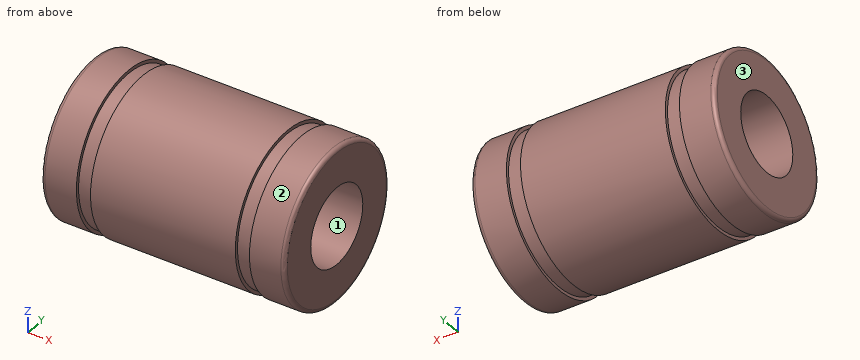
from build123d import *

# Parameters (mm, degrees)
F3_R = 0.3


with BuildPart() as f2:
    # F1 (on Front) → F2 (revolve)
    with BuildSketch(Plane.XZ):
        Polygon((-9.5, 6), (-9.5, 3), (9.5, 3), (9.5, 6), (6.75, 6), (6.75, 5.75), (5.65, 5.75), (5.65, 6), (-5.65, 6), (-5.65, 5.75), (-6.75, 5.75), (-6.75, 6), align=None)
    revolve(axis=Axis((0, 0, 0), (1, 0, 0)))

    # F3
    f3_edges = [f2.edges().sort_by_distance(p)[0] for p in [
        (-9.5, 0, -6),
        (9.5, 0, -6),
    ]]
    fillet(f3_edges, radius=F3_R)


solid = f2.part
Can you work these out from the model? Positions are in its coordinate system, mm. Face numbers are marked on the shaded views. Coordinates: 2 decimals unless noted, no trailing zeros. Order: outer loops, then holes, each group sorted by start corner. A loop starts at its lowest first (then second) coordinate and runs counter-clockwise, first axis right, second up. Notation, with made-up numbers: (-22, -6) - (23, -6) arc R22 ccw to (23, 6) - close; hole circle Ø2 at (79.5, 6). An arc over 180 degrees is marked (long way). Answer as a JSON object with one key per item and string values. Group by question number.
Q1. We'd pull the mould along Z, two halves only. Please class the marked faces 1, 2 and 3: +Z half, -Z half, draft (parallel to the pull), parting line (faces both ways), or undercut.
Q2. Imagine slicing it at D-D (x = -7.5). Please give me the cut outline in (y, z), and give its area (3 significant figures).
Q3. Will these pins go through, and if not, where does the flat tip stop? P1, Ø1, axis at x = -6, z = 4, coming from the -Y side; P2, Ø3.5, axis at y = 0, z = 0, coming from the -X side.
Q4. I need wall thicknesses on line 1 (Z direction, x = -1, y = 0); line 2 (Y direction, x = 6.5, z = 0). Which ranges of each line are inside material? Lowest first, please. Write a range as from..to.
Q5. Imagine slicing it at A-A (y = 0). Please give me the cut outline in (x, z).
Q6. Imagine slicing it at C-C (x = 6). Please give me the cut outline in (y, z), and give its area (3 significant figures).
Determined:
{
 "1": {"face 1": "undercut", "face 2": "parting line", "face 3": "draft"},
 "2": {"outline": "circle Ø12 at (0, 0); hole circle Ø6 at (0, 0)", "area": "84.8 mm2"},
 "3": {"P1": "stops at y = -4.77", "P2": "passes through"},
 "4": {"line 1": "z = -6..-3, 3..6", "line 2": "y = -5.75..-3, 3..5.75"},
 "5": {"outline": "(-9.5, -5.7) arc R0.3 ccw to (-9.2, -6) - (-6.75, -6) - (-6.75, -5.75) - (-5.65, -5.75) - (-5.65, -6) - (5.65, -6) - (5.65, -5.75) - (6.75, -5.75) - (6.75, -6) - (9.2, -6) arc R0.3 ccw to (9.5, -5.7) - (9.5, -3) - (-9.5, -3) - close; (-9.5, 3) - (9.5, 3) - (9.5, 5.7) arc R0.3 ccw to (9.2, 6) - (6.75, 6) - (6.75, 5.75) - (5.65, 5.75) - (5.65, 6) - (-5.65, 6) - (-5.65, 5.75) - (-6.75, 5.75) - (-6.75, 6) - (-9.2, 6) arc R0.3 ccw to (-9.5, 5.7) - close"},
 "6": {"outline": "circle Ø11.5 at (0, 0); hole circle Ø6 at (0, 0)", "area": "75.6 mm2"}
}
